Design review of the part built by this model. Coordinates are the model's own, in mm. Give positions to 0.01 mm unless a question says otherwise; leave off trailing zeros. Loops run counter-clockwise (first coordinate to the right, second up) from the corner with the lowest first, then second, coordinate; pieces in that order, holes last.
from build123d import *

# Parameters (mm, degrees)
SALIENTE_EXTRUIR1_DEPTH = 10


with BuildPart() as part:
    # Croquis1 → Saliente-Extruir1 (new body)
    with BuildSketch(Plane.XY):
        with BuildLine():
            Line((-56.28767918, 206.147542534), (-56.28767918, 26.147542534))
            Line((-56.28767918, 26.147542534), (119.918563855, 26.147542534))
            Line((119.918563855, 26.147542534), (119.918563855, 56.147542534))
            ThreePointArc((119.918563855, 56.147542534), (29.650497915, 108.223742781), (-6.003166727, 206.147542534))
            Line((-6.003166727, 206.147542534), (-56.28767918, 206.147542534))
        make_face()
    extrude(amount=SALIENTE_EXTRUIR1_DEPTH)


solid = part.part
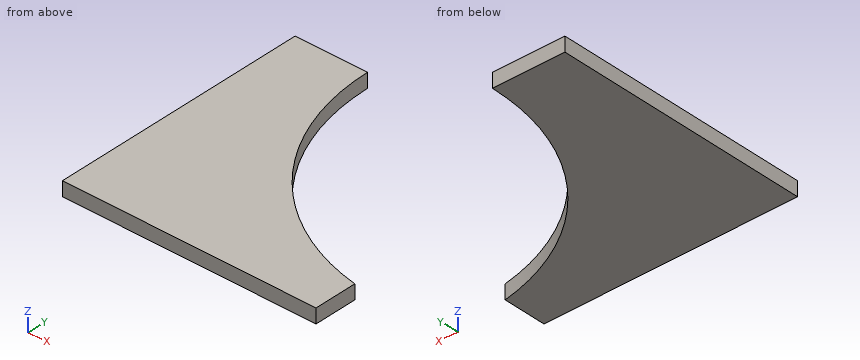
Q1. Wall thickness on line 1 (Y direction, x = 21.5, z = 3); line 2 (X direction, y = 148, z = 4); line 3 (X direction, y = 185, z = 2.5): over which ranges is each line inside the solid? List them lowest first.
Results:
line 1: y = 26.15 to 118.85
line 2: x = -56.29 to 5.53
line 3: x = -56.29 to -4.53
Q2. Insertion check: pin 1 (1 mm diameter, centred on x = 91, z = 6.5, fed in from +Y). The pin has a flat end and moves straight along its axis. Give the tip position at first contact, or say it passes through.
Results:
pin 1: stops at y = 64.44
Q3. Take a section at C-C (x = 59). Give the boundary of the cut face in (y, z), plus the area to 3 significant figures.
Results:
outline: (26.15, 0) - (81.35, 0) - (81.35, 10) - (26.15, 10) - close
area: 552 mm2
Q4. Take a section at A-A (z = 5.5). Give the boundary of the cut face in (x, y).
Results:
outline: (-56.29, 26.15) - (119.92, 26.15) - (119.92, 56.15) arc R152.3 cw to (-6, 206.15) - (-56.29, 206.15) - close
Q5. Take a section at B-B (y = 94). Give the boundary of the cut face in (x, z).
Results:
outline: (-56.29, 0) - (43.25, 0) - (43.25, 10) - (-56.29, 10) - close
